Design review of the part built by this model. Coordinates are the model's own, in mm. Coordinates: 2 decimals unless noted, no trailing zeros. Loops run counter-clockwise (first coordinate to the right, second up) from the corner with the lowest first, then second, coordinate; pieces in that order, holes last. Notation, with made-up numbers: (62.5, 42) -> (110.5, 42) arc R24 ccw to (110.5, 58) -> close; hole circle Ø7 at (-13, -24.75). An arc over 180 degrees is marked (long way). Use a Markdown table: item, result. Add a question column.
Q1. Draft analysis for pull direction X (two halves, no side actions). For faces 1 (the face through (0, -10, 0)), 2 (the face through (0.07, -31.24, 1.5)), 3 (the face through (1, -5, 0)), 4 (the face through (0, -14, -2)), state which applies: pulls with the +X half, pulls with the -X half, needs draft (parallel to the pull), parting line crosses it, or undercut.
Q2. Take a section at D-D on y = -11.5. Write out the cut boundary in (x, z).
Q3. Take a section at A-A on y = -5. Write out the cut boundary in (x, z), plus the area to 3 significant figures.
Q4. For probe 1 along X at (y, z) = (-4, 0); probe 2 along Y at (x, z) = (0.9, -2.05); probe 3 along Z at (x, y) = (0.1, -41), list the stretches that pass through material, from the lowest coordinate up.
Q5. Clearance check with flat-ended pins moving along their axes: pin 1 Ø1 at (x, y) = (0, -42.5) entering from -Z; pin 2 Ø3 at (y, z) = (-25, 0.5) entering from +X; pin 3 Ø1.2 at (x, z) = (0, 0) entering from +Y. State where each tip first meets the part, or that it passes through.
Q6. Take a section at C-C on x = 0. Write out the cut boundary in (y, z).
Q7. Take a section at B-B on z = 0. Write out the cut boundary in (x, y), plus the area to 3 significant figures.
Autodesk Inventor part; units mm, degrees
ref_plane "YZ Plane" through (0, 0, 0) normal (1, 0, 0) x (0, 1, 0)
ref_plane "XZ Plane" through (0, 0, 0) normal (0, 1, 0) x (-1, 0, 0)
ref_plane "XY Plane" through (0, 0, 0) normal (0, 0, 1) x (1, 0, 0)
sketch "Sketch1" plane through (0, 0, 0) normal (1, 0, 0) x (0, 1, 0)
  line L0 (0, 0) -> (-48, 0)
  line L1 (-10, 0) -> (-10, -1)
  line L2 (-10, -1) -> (0, -1)
  line L3 (0, -1) -> (0, -2.5)
  line L4 (0, -2.5) -> (-14, -2.5)
  line L5 (-14, -2.5) -> (-14, -1.5)
  line L6 (-14, -1.5) -> (-48, -1.5)
  line L7 (-48, -1.5) -> (-48, 0)
  point P0 (-10, -0.5)
  point P1 (-14, -2)
  dimension "d0" = 3
  dimension "d1" = 2
  dimension "d2" = 5
  dimension "d3" = 14
  dimension "d4" = 10
  dimension "d6" = 34
revolve "Revolution1" add sketch "Sketch1" angle 360 about axis through (0, 0, 0) along (0, -1, 0)
thread "Thread1"
properties part number "041" material "Stainless Steel, Austenitic"
Answer list:
| question | item | result |
|---|---|---|
| 1 | face 1 | undercut |
| 1 | face 2 | parting line crosses it |
| 1 | face 3 | undercut |
| 1 | face 4 | needs draft |
| 2 | outline | circle Ø5 at (0, 0) |
| 3 | outline | circle Ø5 at (0, 0); hole circle Ø2 at (0, 0) |
| 3 | area | 16.5 mm² |
| 4 | probe 1 | -2.5 to -1, 1 to 2.5 |
| 4 | probe 2 | -14 to 0 |
| 4 | probe 3 | -1.5 to 1.5 |
| 5 | pin 1 | z = -1.5 |
| 5 | pin 2 | x = 1.5 |
| 5 | pin 3 | y = -10 |
| 6 | outline | (-48, -1.5) -> (-14, -1.5) -> (-14, -2.5) -> (0, -2.5) -> (0, -1) -> (-10, -1) -> (-10, 1) -> (0, 1) -> (0, 2.5) -> (-14, 2.5) -> (-14, 1.5) -> (-48, 1.5) -> close |
| 7 | outline | (-2.5, -14) -> (-1.5, -14) -> (-1.5, -48) -> (1.5, -48) -> (1.5, -14) -> (2.5, -14) -> (2.5, 0) -> (1, 0) -> (1, -10) -> (-1, -10) -> (-1, 0) -> (-2.5, 0) -> close |
| 7 | area | 152 mm² |
